Autodesk Inventor part; units mm, degrees
ref_plane "YZ Plane" through (0, 0, 0) normal (1, 0, 0) x (0, 1, 0)
ref_plane "XZ Plane" through (0, 0, 0) normal (0, 1, 0) x (-1, 0, 0)
ref_plane "XY Plane" through (0, 0, 0) normal (0, 0, 1) x (1, 0, 0)
sketch "Sketch2" plane through (0, 0, 0) normal (0, 0, 1) x (1, 0, 0)
  circle A0 centre (-9.8721, 18.0152) radius 2.1844
  circle A1 centre (40.2822, 26.089) radius 2.1844
  circle A2 centre (-26.9412, -26.089) radius 2.1844
  circle A3 centre (-39.6412, 12.011) radius 2.1844
  circle A4 centre (8.0053, 1.7888) radius 2.1844
  circle A5 centre (40.2822, 26.089) radius 6.35
  circle A6 centre (-26.9412, -26.089) radius 6.35
  line L0 (44.2198, 21.1073) -> (-23.0477, -31.1053)
  circle A7 centre (-39.6412, 12.011) radius 6.35
  line L1 (-32.9918, -28.0161) -> (-45.6653, 10.0028)
  line L2 (39.4559, 32.385) -> (-40.7423, 18.2648)
  point P0 (0, 0)
  dimension "d12" = 12.7
  dimension "d13" = 12.7
  dimension "d14" = 12.7
extrude "Extrusion2" add sketch "Sketch2" along normal blind 1.5875 contours A5 L0 A6 L1 A7 L2 | A6 | A7
properties part number "Lbsupportpoly"
For this review, take the finished solid that the model builds, in its own axes (mm). Coordinates: 2 decimals unless noted, no trailing zeros. Order: outer loops, then holes, each group sorted by start corner. A loop starts at its lowest first (then second) coordinate and runs counter-clockwise, first axis right, second up. Notation, with made-up numbers: (-22, -31.5) - (1, -31.5) arc R36 cw to (1, 4.5) - close; hole circle Ø2 at (-18, 19). An arc over 180 degrees is marked (long way). Answer as a JSON object with one key per item and string values. Group by question number.
1. The part is to be moulded in two halves that separate along X. For faces 1 (the flat face through (11.1, -4.6, 0.8)), 2 (the cylindrical face through (-24.86, -26.75, 0.78)), 3 (the flat face through (-11, 8, 0)), 4 (the cylindrical face through (38.55, 27.42, 0.78)), say which applies: pulls with the +X half, pulls with the -X half, needs draft (parallel to the pull), parting line crosses it, or undercut.
2. We need section C-C on y = -12.5. State the section outline as (x, z) points, then the cut area to 3 significant figures.
3. We need section D-D on x = 16.5. State the section outline as (y, z) points, then the cut area to 3 significant figures.
4. For probe 1 along Y at (x, z) = (-11, 0.3); probe 2 along Y at (x, z) = (39, 1); probe 3 along Y at (x, z) = (-6, 0.65), list the stretches that pass through material, from the lowest coordinate up.
5. We need section A-A on x = -39.5. State the section outline as (y, z) points, then the cut area to 3 significant figures.
6. We need section B-B on z = 0.3. State the section outline as (x, y) points (3 decimals).
7. Clearance check with a flat-ended pin moving along its axis: P1, Ø10, axis at x = -25.5, y = -3.5, coming from the -Z side. State where the tip first meets the part, or that it passes through.
Final values:
{
 "1": {"face 1": "pulls with the +X half", "face 2": "undercut", "face 3": "needs draft", "face 4": "undercut"},
 "2": {"outline": "(-38.16, 0) - (0.92, 0) - (0.92, 1.59) - (-38.16, 1.59) - close", "area": "62.0 mm²"},
 "3": {"outline": "(-0.41, 0) - (28.34, 0) - (28.34, 1.59) - (-0.41, 1.59) - close", "area": "45.6 mm²"},
 "4": {"probe 1": "-21.75 to 16.14, 19.89 to 23.5", "probe 2": "17.06 to 24.32, 27.86 to 32.3", "probe 3": "-17.87 to 24.38"},
 "5": {"outline": "(-8.49, 0) - (9.83, 0) - (9.83, 1.59) - (-8.49, 1.59) - close; (14.19, 0) - (18.48, 0) - (18.48, 1.59) - (14.19, 1.59) - close", "area": "35.9 mm²"},
 "6": {"outline": "(-45.665, 10.003) - (-32.992, -28.016) arc R6.35 ccw to (-23.048, -31.105) - (44.22, 21.107) arc R6.35 ccw to (39.456, 32.385) - (-40.742, 18.265) arc R6.35 ccw to start; hole circle Ø4.369 at (-39.641, 12.011); hole circle Ø4.369 at (-26.941, -26.089); hole circle Ø4.369 at (-9.872, 18.015); hole circle Ø4.369 at (8.005, 1.789); hole circle Ø4.369 at (40.282, 26.089)"},
 "7": {"P1": "z = 0"}
}
